```python
from build123d import *

# Parameters (mm, degrees)
SKETCH1_W               = 15.7
SKETCH1_H               = 15.7
BOSS_EXTRUDE1_DEPTH     = 1.5
SKETCH3_R               = 2.4
BOSS_EXTRUDE2_DEPTH     = 1.6
CUT_EXTRUDE1_DEPTH      = 2.1
CUT_EXTRUDE2_DEPTH      = 13.016863151
LPATTERN2_COUNT         = 2
LPATTERN2_PITCH         = 8
LPATTERN2_COUNT_DIR2    = 2
LPATTERN2_PITCH_DIR2    = 8
SKETCH7_R               = 1.5
SKETCH7_R_2             = 1
BOSS_EXTRUDE3_DEPTH     = 1.9
SKETCH10_R              = 1.3
CUT_EXTRUDE3_DEPTH      = 1.7
LPATTERN3_COUNT         = 2
LPATTERN3_PITCH         = 8
LPATTERN3_COUNT_DIR2    = 2
LPATTERN3_PITCH_DIR2    = 8
CUT_EXTRUDE4_DEPTH      = 17.832145471
CUT_EXTRUDE4_DEPTH_BACK = 1.7
FILLET1_R               = 0.2


with BuildPart() as part:
    # Sketch1 → Boss-Extrude1 (new, symmetric)
    with BuildSketch(Plane(origin=(0, 0, 0), x_dir=(1, 0, 0), z_dir=(0, 1, 0))):
        Rectangle(SKETCH1_W, SKETCH1_H)
    extrude(amount=BOSS_EXTRUDE1_DEPTH, both=True)

    # Sketch3 → Boss-Extrude2 (add)
    with BuildSketch(Plane(origin=(0, 1.5, 0), x_dir=(1, 0, 0), z_dir=(0, 1, 0))):
        with Locations(Location((3.95, 3.95, 0), (0, 0, 90))):
            Circle(SKETCH3_R)
    boss_extrude2 = extrude(amount=BOSS_EXTRUDE2_DEPTH)

    # Sketch4 → Cut-Extrude1 (cut)
    with BuildSketch(Plane.XZ.offset(1.5)):
        Polygon((-7.15, 7.15), (-1.15, 7.15), (7.15, -1.15), (7.15, -7.15), (-7.15, -7.15), align=None)
    extrude(amount=-CUT_EXTRUDE1_DEPTH, mode=Mode.SUBTRACT)

    # Sketch6 → Cut-Extrude2 (cut, through all)
    with BuildSketch(Plane.XZ.offset(1.5)):
        Polygon((-0.152943725, 7.85), (7.85, -0.152943725), (7.85, 7.85), align=None)
    extrude(amount=-CUT_EXTRUDE2_DEPTH, mode=Mode.SUBTRACT)

    # LPattern2: Boss-Extrude2 2 × 2, 1 skipped
    with Locations(*[(-i * LPATTERN2_PITCH, 0, j * LPATTERN2_PITCH_DIR2) for i in range(LPATTERN2_COUNT) for j in range(LPATTERN2_COUNT_DIR2) if (i, j) not in ((0, 0), (0, 1))]):
        add(boss_extrude2)

    # Sketch7 → Boss-Extrude3 (add)
    with BuildSketch(Plane.XZ.offset(-0.6)):
        with Locations(Location((0, 0, 0), (0, 0, 270))):
            Circle(SKETCH7_R)
        with Locations(Location((0, 0, 0), (0, 0, 270))):
            Circle(SKETCH7_R_2, mode=Mode.SUBTRACT)
    extrude(amount=BOSS_EXTRUDE3_DEPTH)

    # Sketch10 → Cut-Extrude3 (cut)
    with BuildSketch(Plane.XZ.offset(-0.6)):
        with Locations(Location((-3.95, 3.95, 0), (0, 0, 270))):
            Circle(SKETCH10_R)
    cut_extrude3 = extrude(amount=-CUT_EXTRUDE3_DEPTH, mode=Mode.SUBTRACT)

    # LPattern3: Cut-Extrude3 2 × 2, 1 skipped
    with Locations(*[(j * LPATTERN3_PITCH_DIR2, 0, -i * LPATTERN3_PITCH) for i in range(LPATTERN3_COUNT) for j in range(LPATTERN3_COUNT_DIR2) if (i, j) not in ((0, 0), (0, 1))]):
        add(cut_extrude3, mode=Mode.SUBTRACT)

    # Sketch11 → Cut-Extrude4 (cut, two sides: drawn at the far end of the back side and taken through both)
    with BuildSketch(Plane(origin=(3.848528137, 0, 3.848528137), x_dir=(0.7071067811865478, 0, -0.7071067811865475), z_dir=(0.7071067811865475, 0, 0.7071067811865478)).offset(-CUT_EXTRUDE4_DEPTH_BACK)):
        Polygon((-26.389939678, -34.02340546), (-3.158935778, -1.5), (-1.658935778, 0.6), (1.658935778, 0.6), (3.158935778, -1.5), (26.389939678, -34.02340546), (26.389939678, -113.959666192), (-26.389939678, -113.959666192), align=None)
    extrude(amount=CUT_EXTRUDE4_DEPTH + CUT_EXTRUDE4_DEPTH_BACK, mode=Mode.SUBTRACT)

    # Fillet1
    fillet1_edges = [part.edges().sort_by_distance(p)[0] for p in [
        (4.597308807, 0.6, 2.251219331),
        (1.190559159, -1.5, 5.657968978),
        (5.657968978, -1.5, 1.190559159),
        (2.251219331, 0.6, 4.597308807),
    ]]
    fillet(fillet1_edges, radius=FILLET1_R)


solid = part.part
```
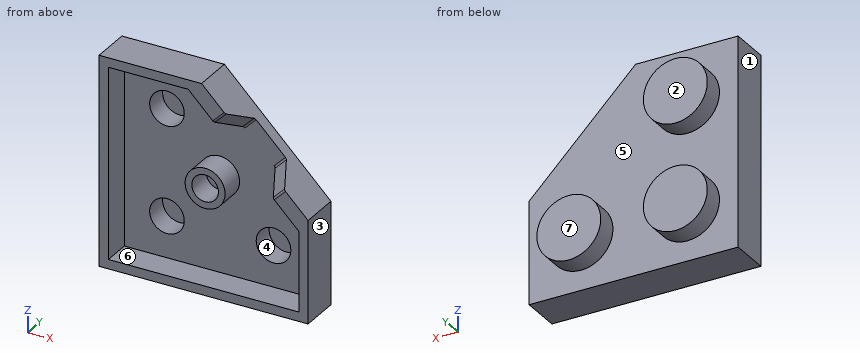
Build history of the part. All positions in model axes, mm. Face numbers are marked on the shaded views. A direction names the side the tool comes from. Round coordinates to 2 decimals unless told otherwise and drop trailing zeros. Write each loop counter-clockwise with the first axis right and the second up, starting at its lowest first coordinate (ties: lowest second). Pieces come first, ordered by that corner, then holes.
1) Band-saw the part on A-A, the plane y = -0.55. List the corners of the cut face in (x, z).
2) Band-saw the part on C-C, the plane z = -4. List the corners of the cut face in (x, y), and give its area (3 significant figures).
3) Band-saw the part on B-B, the plane x = 3.75. List the corners of the cut face in (y, z), and give its area (3 significant figures).
4) Pin check, flat tips, straight feed: pin 1 (1.3 mm diameter, centred on x = 4, z = -4, fed in from -Y); pin 2 (1.2 mm diameter, centred on x = 0, z = 0, fed in from -Y); pin 3 (0.6 mm diameter, centred on y = -0.5, z = 2, fed in from +X). Stop position of each tip, or through.
5) Band-saw the part on D-D, the plane z = 3.5. List the corners of the cut face in (x, y).
6) Mould opens along X. For the marked faces 1, 2, 3 and 4 say: +X half, -X half, draft (parallel to the pull), parting line (faces both ways), or undercut.
7) 3-axis set-ups, long thin cutter, end or side, ignore diameter. For the marked faces 5, 6 and 7: which of +Z, -Z, +X, -X, +Y, -Y reach the whole face in a straight line?
8) Drill centre lines: probe 1 along X at (y, z) = (1.05, -4); probe 2 along X at (y, z) = (1.7, -4.05); probe 3 along Z at (x, y) = (-5.25, 0). Where is each one in solid material? Low to high.
Ans:
1. outline: (-7.85, -7.85) - (7.85, -7.85) - (7.85, -0.15) - (5.6, 2.09) - (4.75, 1.25) - (7.15, -1.15) - (7.15, -7.15) - (-7.15, -7.15) - (-7.15, 7.15) - (-1.15, 7.15) - (1.25, 4.75) - (2.09, 5.6) - (-0.15, 7.85) - (-7.85, 7.85) - close; circle Ø3 at (0, 0); hole circle Ø2 at (0, 0)
2. outline: (-7.85, -1.5) - (-7.15, -1.5) - (-7.15, 0.6) - (-5.25, 0.6) - (-5.25, 2.3) - (-2.65, 2.3) - (-2.65, 0.6) - (2.75, 0.6) - (2.75, 2.3) - (5.35, 2.3) - (5.35, 0.6) - (7.15, 0.6) - (7.15, -1.5) - (7.85, -1.5) - (7.85, 1.5) - (6.35, 1.5) - (6.35, 3.1) - (1.55, 3.1) - (1.55, 1.5) - (-1.65, 1.5) - (-1.65, 3.1) - (-6.45, 3.1) - (-6.45, 1.5) - (-7.85, 1.5) - close
2. area: 23.6 mm2
3. outline: (-1.5, -7.85) - (1.5, -7.85) - (1.5, -6.34) - (3.1, -6.34) - (3.1, -1.56) - (1.5, -1.56) - (1.5, 3.95) - (0.6, 3.95) - (0.6, -2.79) - (2.3, -2.79) - (2.3, -5.31) - (0.6, -5.31) - (0.6, -7.15) - (-1.5, -7.15) - close
3. area: 15.4 mm2
4. pin 1: stops at y = 2.3
4. pin 2: stops at y = 0.6
4. pin 3: stops at x = 6
5. outline: (-7.85, -1.5) - (-7.15, -1.5) - (-7.15, 0.6) - (-5.17, 0.6) - (-5.17, 2.3) - (-2.73, 2.3) - (-2.73, 0.6) - (4.2, 0.6) - (4.2, 1.5) - (-1.71, 1.5) - (-1.71, 3.1) - (-6.39, 3.1) - (-6.39, 1.5) - (-7.85, 1.5) - close
6. face 1: -X half
6. face 2: draft
6. face 3: +X half
6. face 4: undercut
7. face 5: +Y
7. face 6: -Y
7. face 7: +Z, -Z, +X, -X, +Y
8. probe 1: x = -7.85 to -5.25, -2.65 to 2.75, 5.35 to 7.85
8. probe 2: x = -6.45 to -5.25, -2.65 to -1.65, 1.55 to 2.75, 5.35 to 6.35
8. probe 3: z = -7.85 to -7.15, 7.15 to 7.85
